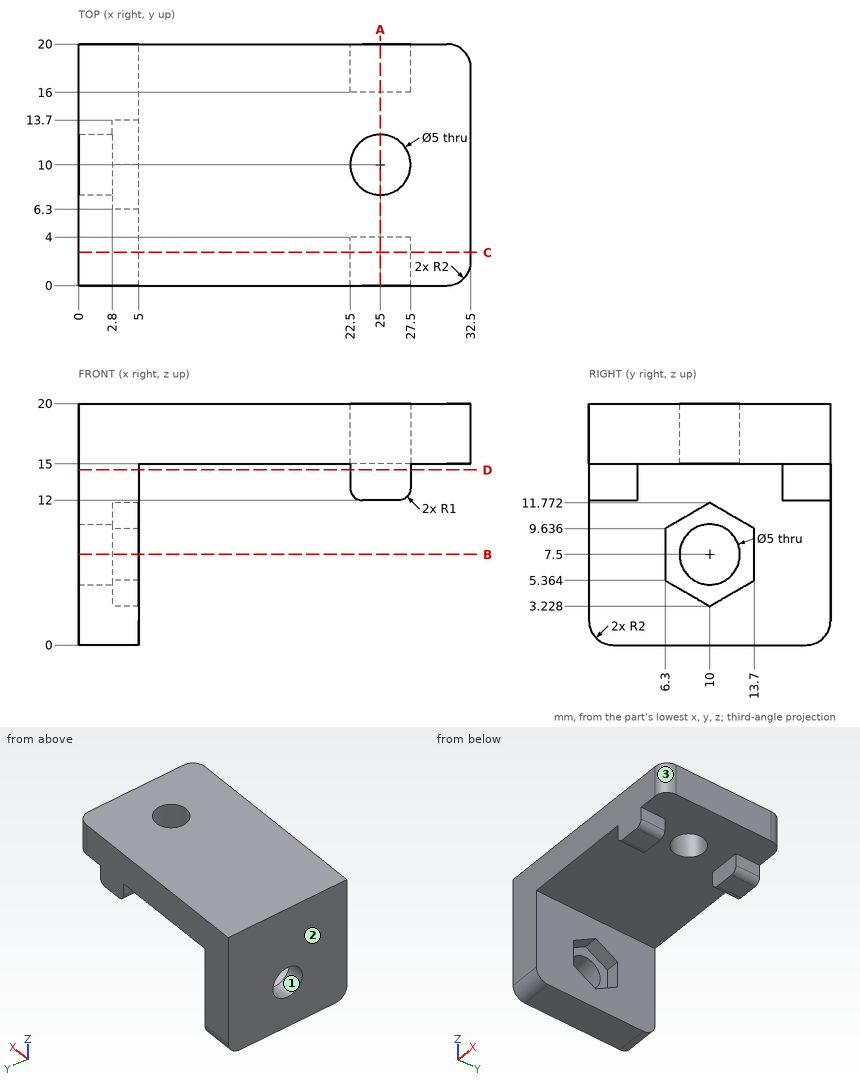
Check sheet for the drawn part. Datum: minimum x, y, z corner. Units: mm. Give positions to 0.01 mm unless a question says otherwise; leave off trailing zeros. Loops run counter-clockwise (first coordinate to the right, second up) from the corner with the lowest first, then second, coordinate; pieces in that order, holes last.
1) Sectioned sample at A-A, the plane x = 25. Enter the section's corners in (y, z).
2) Draft check along Y on the marked faces 1, 2 and 3. Enter one of: pulls with the +Y half, pulls with the -Y half, needs draft (parallel to the pull), parting line crosses it, or undercut.
3) Sectioned sample at B-B, the plane z = 7.5. Enter the section's corners in (x, y).
4) Depth check by flat-ended pin: pin 1 Ø2.5 at (x, y) = (25.5, 17.5) entering from -Z; pin 2 Ø1.6 at (y, z) = (1.5, 13.5) entering from +X; pin 3 Ø3.5 at (y, z) = (8.5, 8) entering from +X. Enter the tip coordinate at first touch or a pass-through.
5) Sectioned sample at D-D, the plane z = 14.5. Enter the section's corners in (x, y), then the cut area to 3 significant figures.
6) Sectioned sample at C-C, the plane y = 2.75. Enter the section's corners in (x, z), then the cut area to 3 significant figures.
7) Thickness scan on line 1 along Y through (x, z) = (25, 17.9); line 2 along Z through (x, y) = (1.85, 10); line 3 along Z through (x, y) = (13, 16). Record the ranges inside material, lowest first.
Answers:
1. outline: (0, 12) - (4, 12) - (4, 15) - (7.5, 15) - (7.5, 20) - (0, 20) - close; (12.5, 15) - (16, 15) - (16, 12) - (20, 12) - (20, 20) - (12.5, 20) - close
2. face 1: undercut
2. face 2: needs draft
2. face 3: pulls with the -Y half
3. outline: (0, 0) - (5, 0) - (5, 6.3) - (2.8, 6.3) - (2.8, 7.5) - (0, 7.5) - close; (0, 12.5) - (2.8, 12.5) - (2.8, 13.7) - (5, 13.7) - (5, 20) - (0, 20) - close
4. pin 1: stops at z = 12
4. pin 2: stops at x = 27.5
4. pin 3: stops at x = 2.8
5. outline: (0, 0) - (5, 0) - (5, 20) - (0, 20) - close; (22.5, 0) - (27.5, 0) - (27.5, 4) - (22.5, 4) - close; (22.5, 16) - (27.5, 16) - (27.5, 20) - (22.5, 20) - close
5. area: 140 mm2
6. outline: (0, 0) - (5, 0) - (5, 15) - (22.5, 15) - (22.5, 13) arc R1 ccw to (23.5, 12) - (26.5, 12) arc R1 ccw to (27.5, 13) - (27.5, 15) - (32.5, 15) - (32.5, 20) - (0, 20) - close
6. area: 252 mm2
7. line 1: y = 0 to 7.5, 12.5 to 20
7. line 2: z = 0 to 5, 10 to 20
7. line 3: z = 15 to 20
